Check sheet for the modelled part. Datum: model origin and axes. Units: mm. A direction names the side the tool comes from. Round coordinates to 2 decimals unless told otherwise and drop trailing zeros. Write each loop counter-clockwise with the first axis right and the second up, starting at its lowest first coordinate (ties: lowest second). Pieces come first, ordered by that corner, then holes. Notation, with made-up numbers: (-25.75, 85.5) - (-21.75, 85.5) arc R10 cw to (-21.75, 95.5) - close; hole circle Ø11 at (13, 66). An arc over 180 degrees is marked (long way). Use one line per item in the form item = value. Start each with the question number.
1) Set-up check for faces 1 (the face through (0.1, -4, 2.5)), 2 (the face through (0, 4, 7)), 3 (the face through (-2.38, -10.74, 1.24)): record each of +Z, -Z, +X, -X, +Y, -Y from which the full face is reachable in a straight line by a thin tool's end or side.
2) Section check B-B (z = 4.5). Record the boundary of the cut face in (x, y).
3) Gauge pin test, flat ends, axial feed: P1, Ø6, axis at y = 5, z = 7.5, coming from the -X side; P2, Ø6, axis at x = 5.5, z = 9, coming from the -Y side; P3, Ø4, axis at y = -3, z = 5.5, coming from the +X side; P4, Ø2, axis at x = 3, y = -2, coming from the +Z side. Record the tip position at first contact, or that the pin passes through.
4) Section check C-C (z = 1). Record the boundary of the cut face in (x, y).
5) Section check A-A (x = 0). Record the boundary of the cut face in (y, z).
6) Scan lines: probe 1 along Z at (x, y) = (5.5, -1); probe 2 along Y at (x, z) = (-2.75, 10.25); probe 3 along X at (y, z) = (-0.5, 1.5). Record each from-to range of solid material in increasing order.
7) Draft check along Y on faces 4 (the face through (0, -2, 2)), 5 (the face through (0, 2, 11)), 6 (the face through (-1.08, -4.88, 2.3)). Enter one of: +Y half, -Y half, draft (parallel to the pull), parting line (faces both ways), or undercut.
from build123d import *

# Parameters (mm, degrees)
F2_DEPTH = 11
F1_R     = 5
F4_DEPTH = 3
F1_R_2   = 11
F6_DEPTH = 2
F7_DEPTH = 2
F8_SIZE  = 0.4
F9_SIZE  = 0.3
F10_SIZE = 0.5


with BuildPart() as f2:
    # F1 (on Top) → F2 (new body)
    with BuildSketch(Plane.XY):
        with BuildLine():
            Line((-4, 0), (4, 0))
            ThreePointArc((4, 0), (0, 4), (-4, 0))
        make_face()
    extrude(amount=F2_DEPTH)

    # F1 (on Top) → F4 (join)
    with BuildSketch(Plane.XY):
        Circle(F1_R)
        with BuildLine():
            ThreePointArc((-4, 0), (0, 4), (4, 0))
            ThreePointArc((4, 0), (0, -4), (-4, 0))
        make_face(mode=Mode.SUBTRACT)
    extrude(amount=F4_DEPTH)

    # F1 (on Top) → F6 (join)
    with BuildSketch(Plane.XY):
        Circle(F1_R_2)
        Circle(F1_R, mode=Mode.SUBTRACT)
    extrude(amount=F6_DEPTH)

    # F1 (on Top) → F7 (join)
    with BuildSketch(Plane.XY):
        with BuildLine():
            ThreePointArc((-4, 0), (0, -4), (4, 0))
            Line((4, 0), (-4, 0))
        make_face()
    extrude(amount=F7_DEPTH)

    # F8
    f8_edges = [f2.edges().sort_by_distance(p)[0] for p in [
        (-5, 0, 3),
    ]]
    chamfer(f8_edges, length=F8_SIZE)

    # F9
    f9_edges = [f2.edges().sort_by_distance(p)[0] for p in [
        (0, 4, 11),
        (0, 0, 11),
    ]]
    chamfer(f9_edges, length=F9_SIZE)

    # F10
    f10_edges = [f2.edges().sort_by_distance(p)[0] for p in [
        (-11, 0, 0),
    ]]
    chamfer(f10_edges, length=F10_SIZE)


solid = f2.part
Results are:
q1.face_1 = +Z
q1.face_2 = +Z, +Y
q1.face_3 = +Z, -Z
q2.outline = (-4, 0) - (4, 0) arc R4 ccw to start
q3.P1 = -3.46
q3.P2 = 0
q3.P3 = through
q3.P4 = 3
q4.outline = circle Ø22 at (0, 0)
q5.outline = (-11, 0.5) - (-10.5, 0) - (10.5, 0) - (11, 0.5) - (11, 2) - (5, 2) - (5, 2.6) - (4.6, 3) - (4, 3) - (4, 10.7) - (3.7, 11) - (0.3, 11) - (0, 10.7) - (0, 2) - (-4, 2) - (-4, 3) - (-4.6, 3) - (-5, 2.6) - (-5, 2) - (-11, 2) - close
q6.probe_1 = 0 to 2
q6.probe_2 = 0 to 2.9
q6.probe_3 = -10.99 to 10.99
q7.face_4 = undercut
q7.face_5 = draft
q7.face_6 = parting line
